Source: CAD feature listing. Evaluate the final solid. Frame: model axes, mm. A direction names the side the tool comes from. Coordinates: 2 decimals unless noted, no trailing zeros. Loops run counter-clockwise (first coordinate to the right, second up) from the corner with the lowest first, then second, coordinate; pieces in that order, holes last.
```python
from build123d import *

# Parameters (mm, degrees)
F0_R     = 12.7
F1_DEPTH = 60.325
F2_R     = 5.08
F3_W     = 52.5957527157
F3_H     = 22.3266
F4_DEPTH = 25.908
F5_DEPTH = 25.4
F6_DEPTH = 25.4
F7_R     = 5.08
F8_R     = 6.35
F9_DEPTH = 25.4


with BuildPart() as f1:
    # F0 (on Front) → F1 (new body)
    with BuildSketch(Plane.XZ):
        with BuildLine():
            ThreePointArc((-45.2591143548, -22.352), (-29.4538635818, -15.8052507731), (-22.9071143548, 0))
            ThreePointArc((-22.9071143548, 0), (-61.0643651279, 15.8052507731), (-45.2591143548, -22.352))
        make_face()
        with Locations((-45.2591143548, 0)):
            Circle(F0_R, mode=Mode.SUBTRACT)
        Polygon((104.8294856452, 0), (71.9872856452, 0), (71.9872856452, -22.352), (171.3012856452, -22.352), (171.3012856452, 0), align=None)
        with BuildLine():
            Line((40.5928856452, 0), (-22.9071143548, 0))
            ThreePointArc((-22.9071143548, 0), (-29.4538635818, -15.8052507731), (-45.2591143548, -22.352))
            Line((-45.2591143548, -22.352), (46.5366914868, -22.352))
            Line((46.5366914868, -22.352), (40.5928856452, 0))
        make_face()
        Polygon((71.9872856452, 0), (40.5928856452, 0), (46.5366914868, -22.352), (71.9872856452, -22.352), align=None)
    extrude(amount=F1_DEPTH)

    # F2
    f2_edges = [f1.edges().sort_by_distance(p)[0] for p in [
        (-22.907114, -30.1625, 0),
        (171.301286, -30.1625, 0),
    ]]
    fillet(f2_edges, radius=F2_R)

    # F3 (on face) → F4 (cut, symmetric)
    with BuildSketch(Plane.XY):
        with Locations((-44.5994644167, -30.1625)):
            Rectangle(F3_W, F3_H)
    extrude(amount=F4_DEPTH, both=True, mode=Mode.SUBTRACT)

    # F0 (on Front) → F5 (join)
    with BuildSketch(Plane.XZ):
        with BuildLine():
            ThreePointArc((85.7794856452, 34.798), (82.2053010067, 16.0823576341), (71.9872856452, 0))
            Line((71.9872856452, 0), (104.8294856452, 0))
            Line((104.8294856452, 0), (104.8294856452, 34.798))
            Line((104.8294856452, 34.798), (85.7794856452, 34.798))
        make_face()
    extrude(amount=F5_DEPTH)

    # F0 (on Front) → F6 (cut)
    with BuildSketch(Plane.XZ):
        Polygon((71.9872856452, 0), (40.5928856452, 0), (46.5366914868, -22.352), (71.9872856452, -22.352), align=None)
    extrude(amount=F6_DEPTH, mode=Mode.SUBTRACT)

    # F7
    f7_edges = [f1.edges().sort_by_distance(p)[0] for p in [
        (104.829486, -12.7, 0),
        (104.829486, -12.7, 34.798),
    ]]
    fillet(f7_edges, radius=F7_R)

    # F8 (on face) → F9 (cut)
    with BuildSketch(Plane.XY):
        with Locations((147.1694111824, -47.9711517692)):
            Circle(F8_R)
    extrude(amount=-F9_DEPTH, mode=Mode.SUBTRACT)


solid = f1.part
```
Q1. Section query B-B on y = -22.5. Return the cut outline in (x, z).
Q2. Reachability of faces 1 (the flat face through (75, -30, 0)), 2 (the flat face through (104.829, -13, 17)), 3 (the flat face through (95, -25.4, 18)), 4 (the flat face through (-18.302, -30, -11)) from +Z, -Z, +X, -X, +Y, -Y: full face, straight path, thin tool, end or side. Return the list, or none.
Q3. First-contact query: pin 1 Ø13.5 at (x, z) = (-44, 6) entering from +Y; pin 2 Ø16.5 at (x, y) = (147.17, -47.97) entering from +Z; pin 3 Ø1.5 at (y, z) = (-10.5, -3) entering from +X; pin 4 Ø10 at (x, y) = (-41, -51.5) entering from +Z. Flat tips, straight axial feed; report the tip coordinate or a pass-through.
Q4. Section query A-A on y = -52. Return the cut outline in (x, z), then the cut area to 3 significant figures.
Q5. Material intervals for line 1 along X through (y, z) = (-6, -9.5); line 2 along Z through (x, y) = (-45.5, -54); line 3 along Z through (x, y) = (59, -29.5), sorted ascending.
Q6. Section query C-C on z = 17.5. Return the cut outline in (x, y) (3 decimals).
Q7. Section query D-D on x = 92.5. Return the cut outline in (y, z) (3 decimals).
Q8. Draft query along Y for faces 5 (the cylindrical face through (103.38, -12.88, 33.27)), 6 (the flat face through (-32, -41.326, 0)), 7 (the flat face through (-11, 0, -5)). Return one class per face: released by +Y, released by -Y, zero draft, split by the parting line, or undercut.
Resolved:
1. outline: (-18.3, -22.35) - (46.54, -22.35) - (40.59, 0) - (-18.3, 0) - close; (71.99, -22.35) - (171.3, -22.35) - (171.3, -5.08) arc R5.08 ccw to (166.22, 0) - (109.91, 0) arc R5.08 cw to (104.83, 5.08) - (104.83, 29.72) arc R5.08 ccw to (99.75, 34.8) - (85.78, 34.8) arc R50.8 cw to (71.99, 0) - close
2. face 1: +Z, -Y
2. face 2: +Z, +X, +Y, -Y
2. face 3: +Z, +X, -X, -Y
2. face 4: +Z, -Z, -X
3. pin 1: stops at y = 0
3. pin 2: stops at z = 0
3. pin 3: stops at x = 171.12
3. pin 4: stops at z = 22.35
4. outline: (-45.26, -22.35) - (142.26, -22.35) - (142.26, 0) - (-18.3, 0) arc R5.08 cw to (-23.29, 4.14) arc R22.35 ccw (long way) to start; (152.08, -22.35) - (171.3, -22.35) - (171.3, -5.08) arc R5.08 ccw to (166.22, 0) - (152.08, 0) - close; hole circle Ø25.4 at (-45.26, 0)
4. area: 5,290 mm2
5. line 1: x = -65.49 to -53.69, -36.83 to 43.12, 71.99 to 171.3
5. line 2: z = -22.35 to -12.7, 12.7 to 22.35
5. line 3: z = -22.35 to 0
6. outline: (-59.165, -60.325) - (-31.354, -60.325) - (-31.354, -41.326) - (-59.165, -41.326) - close; (-59.165, -18.999) - (-31.354, -18.999) - (-31.354, 0) - (-59.165, 0) - close; (82.743, -25.4) - (104.829, -25.4) - (104.829, 0) - (82.743, 0) - close
7. outline: (-60.325, -22.352) - (0, -22.352) - (0, 34.798) - (-25.4, 34.798) - (-25.4, 0) - (-60.325, 0) - close
8. face 5: zero draft
8. face 6: undercut
8. face 7: released by +Y
